Autodesk Inventor part; units mm, degrees
ref_plane "YZ Plane" through (0, 0, 0) normal (1, 0, 0) x (0, 1, 0)
ref_plane "XZ Plane" through (0, 0, 0) normal (0, 1, 0) x (-1, 0, 0)
ref_plane "XY Plane" through (0, 0, 0) normal (0, 0, 1) x (1, 0, 0)
sketch "Эскиз1" plane through (0, 0, 0) normal (0, 0, 1) x (1, 0, 0)
  line L0 (-12.5, 3) -> (12.5, 3)
  line L1 (12.5, 3) -> (12.5, -3)
  line L2 (-12.5, -3) -> (-12.5, 3)
  arc A0 (10.5784, -3) -> (4.9216, -3) centre (7.75, -4) ccw
  arc A1 (-3.1193, -3) -> (-11.3807, -3) centre (-7.25, -4) ccw
  line L3 (12.5, -3) -> (10.5784, -3)
  line L4 (4.9216, -3) -> (-3.1193, -3)
  line L5 (-11.3807, -3) -> (-12.5, -3)
  point P0 (0, 0)
  point P1 (-12.5, 0)
  point P2 (0, 3)
  dimension "d0" = 25
  dimension "d1" = 6
  dimension "d2" = 6
  dimension "d3" = 8.5
  dimension "d7" = 5.25
  dimension "d8" = 15
extrude "Выдавливание1" add sketch "Эскиз1" along normal blind 10
sketch "Эскиз2" plane through (-12.5, 3, 0) normal (0, 1, 0) x (1, 0, 0)
  point P0 (12.5, 0)
  point P1 (12.5, -5)
hole "Отверстие1" at (0, 3, 5) direction (0, -1, 0) diameter 3 end through all
properties part number "Крепление кабеля"
Here's how the part is built. I have some questions about the finished solid (model axes, mm). Round coordinates to 2 decimals unless told otherwise and drop trailing zeros. Order: outer loops, then holes, each group sorted by start corner. A loop starts at its lowest first (then second) coordinate and runs counter-clockwise, first axis right, second up. Notation, with made-up numbers: M -23,-5.5 L -15,-5.5 A22 ccw -15,25.5 Z; hole C -14,25 d7. An arc over 180 degrees is marked long. One line per question, with ' | ' between items.
1) I need wall thicknesses on line 1 along X through (y, z) = (-1.25, 8); line 2 along X through (y, z) = (-1.5, 1); line 3 along X through (y, z) = (1.5, 5). Which ranges of each line are inside material? Lowest first, please.
Working result:
line 1: -12.5 to -10.49, -4.01 to 6.55, 8.95 to 12.5 | line 2: -12.5 to -10.69, -3.81 to 6.09, 9.41 to 12.5 | line 3: -12.5 to -1.5, 1.5 to 12.5
2) I want a section at C-C, the plane y = -1.25. Write out the boundary of the cut face in (x, z).
Working result:
outline: M -12.5,0 L -10.49,0 L -10.49,10 L -12.5,10 Z; M -4.01,0 L 6.55,0 L 6.55,10 L -4.01,10 Z; M 8.95,0 L 12.5,0 L 12.5,10 L 8.95,10 Z; hole C 0,5 d3
3) I want a section at B-B, the plane z = 5. Write out the boundary of the cut face in (x, y), then the cut area to 3 significant figures.
Working result:
outline: M -12.5,-3 L -11.38,-3 A4.25 cw -3.12,-3 L -1.5,-3 L -1.5,3 L -12.5,3 Z; M 1.5,-3 L 4.92,-3 A3 cw 10.58,-3 L 12.5,-3 L 12.5,3 L 1.5,3 Z | area: 104 mm²
4) If we mould it in two halves opening along X, with no side actions, what happens to faces 1 (the face through (-12.5, 0, 5)), 2 (the face through (7.7, -1, 4.9)), 3 (the face through (0, 0, 0))? For each: +X half, -X half, draft (parallel to the pull), parting line (faces both ways), or undercut.
Working result:
face 1: -X half | face 2: undercut | face 3: draft
5) For pin 1 Ø2.5 at (x, z) = (0, 5) entering from +Y, with a flat end and sliding along its axis, tell me the tip position at first contact or that it passes through.
Working result:
pin 1: through
6) I want a section at A-A, the plane x = 0. Write out the boundary of the cut face in (y, z), then the cut area to 3 significant figures.
Working result:
outline: M -3,0 L 3,0 L 3,3.5 L -3,3.5 Z; M -3,6.5 L 3,6.5 L 3,10 L -3,10 Z | area: 42.0 mm²
7) I want a section at D-D, the plane y = 2.75. Write out the boundary of the cut face in (x, z).
Working result:
outline: M -12.5,0 L 12.5,0 L 12.5,10 L -12.5,10 Z; hole C 0,5 d3
